Part print with two shaded views. Sizes in mm from the minimum x, y, z corner. Give positions to 0.01 mm unless a question says otherwise; leave off trailing zeros. Order: outer loops, then holes, each group sorted by start corner. A loop starts at its lowest first (then second) coordinate and runs counter-clockwise, first axis right, second up. Notation, with made-up numbers: M 69,-34 L 112,-34 A4 cw 112,-29 Z; hole C 51.25,27 d6. An arc over 180 degrees is marked long. Return JSON: item names as keys, results as strings. Group by question number.
1. Slice it at C-C on y = 38. List the corners of the cut face in (x, z), then the cut area to 3 significant figures.
2. Slice it at D-D on x = 29. List the corners of the cut face in (y, z).
3. Slice it at A-A on y = 2.5. List the corners of the cut face in (x, z).
4. Wall check: probe 1 along X at (y, z) = (77.5, 2.45); probe 2 along Y at (x, z) = (66.5, 2.55); probe 3 along X at (y, z) = (55, 2.65). Give the ranges that are in metal, low to high. Write a range as [from, to].
5. Slice it at B-B on x = 18.5. List the corners of the cut face in (y, z), then the cut area to 3 significant figures.
6. Pin check, flat tips, straight feed: pin 1 (4 mm diameter, centred on x = 18.5, y = 77.5, fed in from -Z); pin 2 (1.5 mm diameter, centred on y = 31.5, z = 2, fed in from -X). Stop position of each tip, or through.
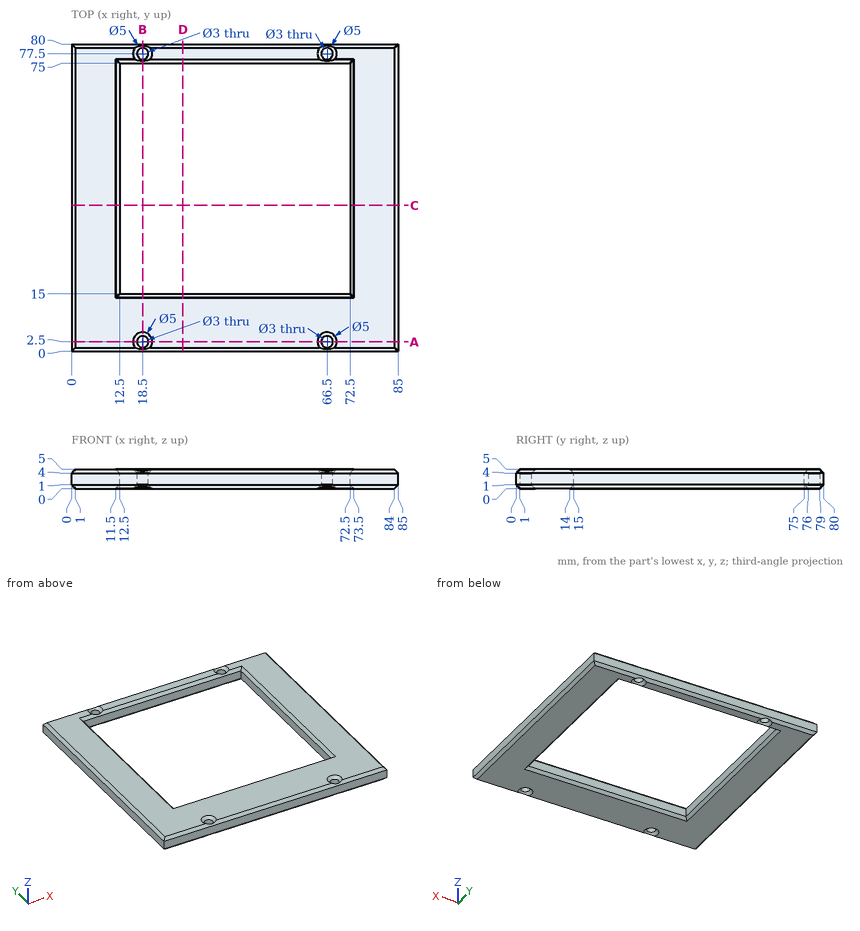
Result:
{
 "1": {"outline": "M 0,1 L 1,0 L 11.5,0 L 12.5,1 L 12.5,4 L 11.5,5 L 1,5 L 0,4 Z; M 72.5,1 L 73.5,0 L 84,0 L 85,1 L 85,4 L 84,5 L 73.5,5 L 72.5,4 Z", "area": "121 mm2"},
 "2": {"outline": "M 0,1 L 1,0 L 14,0 L 15,1 L 15,4 L 14,5 L 1,5 L 0,4 Z; M 75,1 L 76,0 L 79,0 L 80,1 L 80,4 L 79,5 L 76,5 L 75,4 Z"},
 "3": {"outline": "M 0,1 L 1,0 L 16,0 L 17,1 L 17,4 L 16,5 L 1,5 L 0,4 Z; M 20,1 L 21,0 L 64,0 L 65,1 L 65,4 L 64,5 L 21,5 L 20,4 Z; M 68,1 L 69,0 L 84,0 L 85,1 L 85,4 L 84,5 L 69,5 L 68,4 Z"},
 "4": {"probe 1": "x = [0, 17], [20, 65], [68, 85]", "probe 2": "y = [0, 1], [4, 15], [75, 76], [79, 80]", "probe 3": "x = [0, 12.5], [72.5, 85]"},
 "5": {"outline": "M 0,1 L 0.5,0.5 L 1,1 L 1,4 L 0.5,4.5 L 0,4 Z; M 4,1 L 5,0 L 14,0 L 15,1 L 15,4 L 14,5 L 5,5 L 4,4 Z; M 75,1 L 75.5,0.5 L 76,1 L 76,4 L 75.5,4.5 L 75,4 Z; M 79,1 L 79.5,0.5 L 80,1 L 80,4 L 79.5,4.5 L 79,4 Z", "area": "63.5 mm2"},
 "6": {"pin 1": "stops at z = 0.5", "pin 2": "stops at x = 0"}
}
